from build123d import *

# Parameters (mm, degrees)
SKETCH_1_R           = 1.75
EXTRUDE_3_DEPTH      = 3
EXTRUDE_4_DEPTH      = 15
SKETCH_3_R           = 1
CUT_EXTRUDE_5_DEPTH  = 7.5
SKETCH_8_R           = 0.85
CUT_EXTRUDE_8_DEPTH  = 9
SKETCH_10_R          = 0.85
CUT_EXTRUDE_9_DEPTH  = 9
SKETCH_11_R          = 0.85
CUT_EXTRUDE_10_DEPTH = 9
SKETCH_12_R          = 0.85
CUT_EXTRUDE_11_DEPTH = 9
SKETCH_13_R          = 1.25
SKETCH_13_R_2        = 0.85
EXTRUDE_5_DEPTH      = 5
SKETCH_14_R          = 1.25
SKETCH_14_R_2        = 0.85
EXTRUDE_6_DEPTH      = 5
SKETCH_15_R          = 1.25
SKETCH_15_R_2        = 0.85
EXTRUDE_7_DEPTH      = 5
SKETCH_16_R          = 1.25
SKETCH_16_R_2        = 0.85
EXTRUDE_8_DEPTH      = 5
SKETCH_17_R          = 1.25
SKETCH_17_R_2        = 1
EXTRUDE_9_DEPTH      = 5


with BuildPart() as part:
    # 草图1 → 凸台-拉伸3 (new body)
    with BuildSketch(Plane.XY):
        with BuildLine():
            Line((-18, -25), (18, -25))
            ThreePointArc((18, -25), (22.949747468, -22.949747468), (25, -18))
            Line((25, -18), (25, 18))
            ThreePointArc((25, 18), (22.949747468, 22.949747468), (18, 25))
            Line((18, 25), (-18, 25))
            ThreePointArc((-18, 25), (-22.949747468, 22.949747468), (-25, 18))
            Line((-25, 18), (-25, -18))
            ThreePointArc((-25, -18), (-22.949747468, -22.949747468), (-18, -25))
        make_face()
        with Locations((20, 20)):
            Circle(SKETCH_1_R, mode=Mode.SUBTRACT)
        with Locations((-20, 20)):
            Circle(SKETCH_1_R, mode=Mode.SUBTRACT)
        with Locations((-20, -20)):
            Circle(SKETCH_1_R, mode=Mode.SUBTRACT)
        with Locations((20, -20)):
            Circle(SKETCH_1_R, mode=Mode.SUBTRACT)
    extrude(amount=EXTRUDE_3_DEPTH)

    # 草图2 → 凸台-拉伸4 (add)
    with BuildSketch(Plane(origin=(0, 0, 0), x_dir=(-1, 0, 0), z_dir=(0, 0, -1))):
        Polygon((9.814954576, -17), (19.629909152, 0), (9.814954576, 17), (-9.814954576, 17), (-19.629909152, 0), (-9.814954576, -17), align=None)
    extrude(amount=EXTRUDE_4_DEPTH)

    # 草图3 → 切除-拉伸5 (cut)
    with BuildSketch(Plane(origin=(0, 0, -15), x_dir=(-1, 0, 0), z_dir=(0, 0, -1))):
        with Locations((-4.815101245, 8.34)):
            Circle(SKETCH_3_R)
        with Locations((4.815101245, 8.34)):
            Circle(SKETCH_3_R)
        with Locations((4.815101245, -8.34)):
            Circle(SKETCH_3_R)
        with Locations((-4.815101245, -8.34)):
            Circle(SKETCH_3_R)
    extrude(amount=-CUT_EXTRUDE_5_DEPTH, mode=Mode.SUBTRACT)

    # 草图8 → 切除-拉伸8 (cut)
    with BuildSketch(Plane(origin=(14.722431864, 8.5, 0), x_dir=(0, 0, -1), z_dir=(0.866025404, 0.5, 0))):
        with Locations((10, 4.814954576)):
            Circle(SKETCH_8_R)
    extrude(amount=-CUT_EXTRUDE_8_DEPTH, mode=Mode.SUBTRACT)

    # 草图10 → 切除-拉伸9 (cut)
    with BuildSketch(Plane(origin=(-14.722431864, 8.5, 0), x_dir=(0, 0, 1), z_dir=(-0.866025404, 0.5, 0))):
        with Locations((-10, 4.814954576)):
            Circle(SKETCH_10_R)
    extrude(amount=-CUT_EXTRUDE_9_DEPTH, mode=Mode.SUBTRACT)

    # 草图11 → 切除-拉伸10 (cut)
    with BuildSketch(Plane(origin=(-14.722431864, -8.5, 0), x_dir=(0, 0, 1), z_dir=(-0.866025404, -0.5, 0))):
        with Locations((-10, -4.814954576)):
            Circle(SKETCH_11_R)
    extrude(amount=-CUT_EXTRUDE_10_DEPTH, mode=Mode.SUBTRACT)

    # 草图12 → 切除-拉伸11 (cut)
    with BuildSketch(Plane(origin=(14.722431864, -8.5, 0), x_dir=(0, 0, -1), z_dir=(0.866025404, -0.5, 0))):
        with Locations((10, -4.814954576)):
            Circle(SKETCH_12_R)
    extrude(amount=-CUT_EXTRUDE_11_DEPTH, mode=Mode.SUBTRACT)

    # 草图13 → 凸台-拉伸5 (add)
    with BuildSketch(Plane(origin=(14.722431864, 8.5, 0), x_dir=(0, 0, -1), z_dir=(0.866025404, 0.5, 0))):
        with Locations((10, 4.814954576)):
            Circle(SKETCH_13_R)
        with Locations((10, 4.814954576)):
            Circle(SKETCH_13_R_2, mode=Mode.SUBTRACT)
    extrude(amount=EXTRUDE_5_DEPTH)

    # 草图14 → 凸台-拉伸6 (add)
    with BuildSketch(Plane(origin=(-14.722431864, 8.5, 0), x_dir=(0, 0, 1), z_dir=(-0.866025404, 0.5, 0))):
        with Locations((-10, 4.814954576)):
            Circle(SKETCH_14_R)
        with Locations((-10, 4.814954576)):
            Circle(SKETCH_14_R_2, mode=Mode.SUBTRACT)
    extrude(amount=EXTRUDE_6_DEPTH)

    # 草图15 → 凸台-拉伸7 (add)
    with BuildSketch(Plane(origin=(-14.722431864, -8.5, 0), x_dir=(0, 0, 1), z_dir=(-0.866025404, -0.5, 0))):
        with Locations((-10, -4.814954576)):
            Circle(SKETCH_15_R)
        with Locations((-10, -4.814954576)):
            Circle(SKETCH_15_R_2, mode=Mode.SUBTRACT)
    extrude(amount=EXTRUDE_7_DEPTH)

    # 草图16 → 凸台-拉伸8 (add)
    with BuildSketch(Plane(origin=(14.722431864, -8.5, 0), x_dir=(0, 0, -1), z_dir=(0.866025404, -0.5, 0))):
        with Locations((10, -4.814954576)):
            Circle(SKETCH_16_R)
        with Locations((10, -4.814954576)):
            Circle(SKETCH_16_R_2, mode=Mode.SUBTRACT)
    extrude(amount=EXTRUDE_8_DEPTH)

    # 草图17 → 凸台-拉伸9 (add)
    with BuildSketch(Plane(origin=(0, 0, -15), x_dir=(-1, 0, 0), z_dir=(0, 0, -1))):
        with Locations((4.815101245, 8.34)):
            Circle(SKETCH_17_R)
        with Locations((4.815101245, 8.34)):
            Circle(SKETCH_17_R_2, mode=Mode.SUBTRACT)
        with Locations((-4.815101245, 8.34)):
            Circle(SKETCH_17_R)
        with Locations((-4.815101245, 8.34)):
            Circle(SKETCH_17_R_2, mode=Mode.SUBTRACT)
        with Locations((-4.815101245, -8.34)):
            Circle(SKETCH_17_R)
        with Locations((-4.815101245, -8.34)):
            Circle(SKETCH_17_R_2, mode=Mode.SUBTRACT)
        with Locations((4.815101245, -8.34)):
            Circle(SKETCH_17_R)
        with Locations((4.815101245, -8.34)):
            Circle(SKETCH_17_R_2, mode=Mode.SUBTRACT)
    extrude(amount=EXTRUDE_9_DEPTH)


solid = part.part
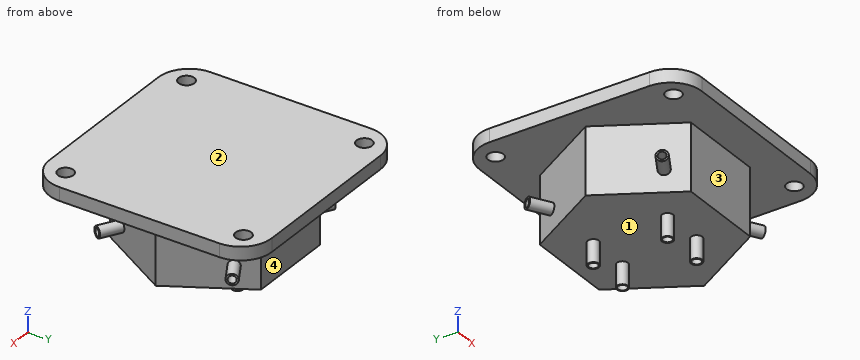
Model file for the job. Use its own axes, mm. Face numbers are marked on the shaded views. A direction names the side the tool comes from. Round coordinates to 2 decimals unless told otherwise and drop trailing zeros. Loops run counter-clockwise (first coordinate to the right, second up) from the corner with the lowest first, then second, coordinate; pieces in that order, holes last.
1. Band-saw the part on A-A, the plane z = -17. List the corners of the cut face in (x, y).
Check values:
outline: circle Ø2.5 at (-4.82, -8.34); circle Ø2.5 at (-4.82, 8.34); circle Ø2.5 at (4.82, -8.34); circle Ø2.5 at (4.82, 8.34); hole circle Ø2 at (-4.82, -8.34); hole circle Ø2 at (-4.82, 8.34); hole circle Ø2 at (4.82, -8.34); hole circle Ø2 at (4.82, 8.34)
2. Band-saw the part on B-B, the plane y = -20. List the corners of the cut face in (x, z), and give its area (3 significant figures).
Check values:
outline: (-24.71, 0) - (-21.75, 0) - (-21.75, 3) - (-24.71, 3) - close; (-18.25, 0) - (18.25, 0) - (18.25, 3) - (-18.25, 3) - close; (21.75, 0) - (24.71, 0) - (24.71, 3) - (21.75, 3) - close
area: 127 mm2
3. Band-saw the part on C-C, the plane z = -13.25. List the corners of the cut face in (x, y).
Check values:
outline: (-19.63, 0) - (-9.81, -17) - (9.81, -17) - (19.63, 0) - (9.81, 17) - (-9.81, 17) - close; hole circle Ø2 at (-4.82, -8.34); hole circle Ø2 at (-4.82, 8.34); hole circle Ø2 at (4.82, -8.34); hole circle Ø2 at (4.82, 8.34)
4. Wall check: probe 1 along Z at (x, y) = (-14.5, 14); probe 2 along Z at (x, y) = (-6, 9); probe 3 along Y at (x, z) = (-4, -9). Give the ranges that are in metal, low to high.
Check values:
probe 1: z = -11.25 to -10.85, -9.15 to -8.75, 0 to 3
probe 2: z = -15 to -10.85, -9.15 to 3
probe 3: y = -17 to -8.92, -7.76 to 7.76, 8.92 to 17
5. Drop flat-ended pins along their axis: P1, Ø2.5, axis at x = 4.82, y = 8.34, coming from the -Z side; P2, Ø1, axis at x = 13.5, z = -14, coming from the -Y side; P3, Ø2, axis at x = -20, y = -20, coming from the +Z side; P4, Ø4.5, axis at x = -20, y = 20, coming from the -Z side. Give the stop position or say it passes through.
Check values:
P1: stops at z = -20
P2: stops at y = -11.48
P3: passes through
P4: stops at z = 0
6. Band-saw the part on D-D, the plane x = -19. List the corners of the cut face in (y, z), and give its area (3 significant figures).
Check values:
outline: (-24.93, 0) - (-21.44, 0) - (-21.44, 3) - (-24.93, 3) - close; (-18.56, 0) - (-1.09, 0) - (-1.09, -15) - (1.09, -15) - (1.09, 0) - (18.56, 0) - (18.56, 3) - (-18.56, 3) - close; (21.44, 0) - (24.93, 0) - (24.93, 3) - (21.44, 3) - close
area: 165 mm2
7. Tool access for the marked faces 1, 2, 3 and 4: list every direction of +Z, -Z, +X, -X, +Y, -Y with a clear straight run to the whole face (end or side of a thin tool).
Check values:
face 1: -Z
face 2: +Z, +X, -X, +Y, -Y
face 3: -Z, +X, -X, -Y
face 4: -Z, +X, -X, +Y
